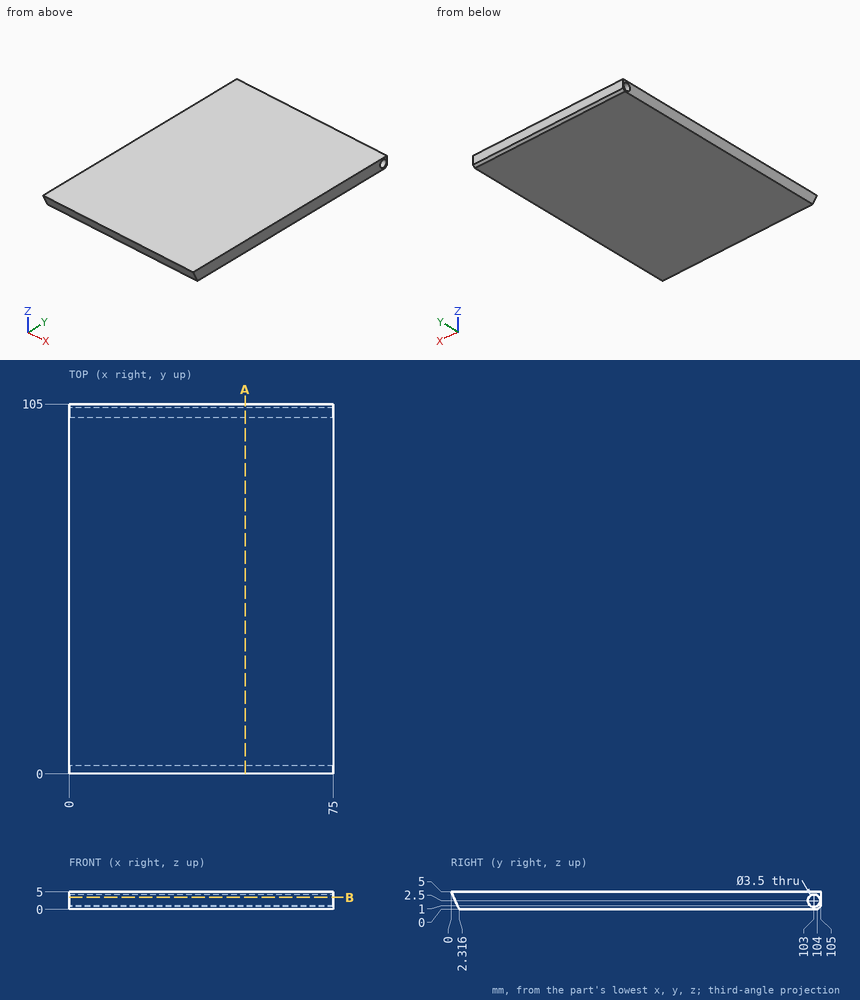
Check sheet for the drawn part. Datum: minimum x, y, z corner. Units: mm. Coordinates: 2 decimals unless noted, no trailing zeros. Loops run counter-clockwise (first coordinate to the right, second up) from the corner with the lowest first, then second, coordinate; pieces in that order, holes last. Notation, with made-up numbers: (55, 18) -> (94, 18) arc R23 ccw to (94, 27) -> close; hole circle Ø3 at (87.5, 9.5). An arc over 180 degrees is marked (long way). Answer as a JSON object with one key per item and string values. Group by question number.
Item 1: Sectioned sample at B-B on z = 3.45. Record the boundary of the cut face in (x, y).
Item 2: Depth check by flat-ended pin: pin 1 (1.5 mm diameter, centred on x = 53.5, z = 3, fed in from -Y); pin 2 (3 mm diameter, centred on y = 103, z = 2.5, fed in from +X). Enter the tip coordinate at first touch or a pass-through.
Item 3: Scan lines: probe 1 along Y at (x, z) = (22.5, 3.85) (1 decimal); probe 2 along Y at (x, z) = (33, 1.5) (1 decimal); probe 3 along Y at (x, z) = (40.5, 0.5) (1 decimal). Record each from-to range of solid material in increasing order.
Item 4: Sectioned sample at A-A on x = 50. Record the boundary of the cut face in (y, z), plus the area to 3 significant figures.
Evaluation:
{
 "1": {"outline": "(0, 0.72) -> (75, 0.72) -> (75, 101.53) -> (0, 101.53) -> close; (0, 104.47) -> (75, 104.47) -> (75, 105) -> (0, 105) -> close"},
 "2": {"pin 1": "stops at y = 0.58", "pin 2": "passes through"},
 "3": {"probe 1": "y = 0.5 to 101.9, 104.1 to 105", "probe 2": "y = 1.6 to 101.6, 104.4 to 105", "probe 3": "y = 2.1 to 104.5"},
 "4": {"outline": "(0, 5) -> (2.32, 0) -> (104, 0) -> (105, 1) -> (105, 5) -> close; hole circle Ø3.5 at (103, 2.5)", "area": "509 mm²"}
}
